```python
from build123d import *

# Parameters (mm, degrees)
F0_R     = 1.5875
F1_DEPTH = 1.6256


with BuildPart() as f1:
    # F0 (on Top) → F1 (new body)
    with BuildSketch(Plane.XY):
        with BuildLine():
            Line((-7.3025, -23.9776), (7.3025, -23.9776))
            ThreePointArc((7.3025, -23.9776), (8.425032, -23.512632), (8.89, -22.3901))
            Line((8.89, -22.3901), (8.89, 22.3901))
            ThreePointArc((8.89, 22.3901), (8.425032, 23.512632), (7.3025, 23.9776))
            Line((7.3025, 23.9776), (-7.3025, 23.9776))
            ThreePointArc((-7.3025, 23.9776), (-8.425032, 23.512632), (-8.89, 22.3901))
            Line((-8.89, 22.3901), (-8.89, -22.3901))
            ThreePointArc((-8.89, -22.3901), (-8.425032, -23.512632), (-7.3025, -23.9776))
        make_face()
        with Locations((0, -20.6756)):
            Circle(F0_R, mode=Mode.SUBTRACT)
        with Locations((0, 20.6756)):
            Circle(F0_R, mode=Mode.SUBTRACT)
    extrude(amount=-F1_DEPTH)


solid = f1.part
```
The listing builds one solid part. Answer for the finished solid, in the listing's coordinates (mm). Give positions to 0.01 mm unless a question says otherwise; leave off trailing zeros. Order: outer loops, then holes, each group sorted by start corner. A loop starts at its lowest first (then second) coordinate and runs counter-clockwise, first axis right, second up.
Item 1: For a pull along Y with two mould halves and no side action, classify faces 1 (the face through (-0.344, 19.126, -0.801)), 2 (the face through (0.853, -19.337, -0.801)), 3 (the face through (-8.89, 0, -1)), 4 (the face through (0, 23.978, -1)) as pulls with the +Y half, pulls with the -Y half, needs draft (parallel to the pull), parting line crosses it, or undercut.
From the geometry:
face 1: undercut
face 2: undercut
face 3: needs draft
face 4: pulls with the +Y half
Item 2: The part is cut by section A-A, the plane x = 0. Give the vertices of the cut face in (y, z).
From the geometry:
outline: (-23.98, -1.63) - (-22.26, -1.63) - (-22.26, 0) - (-23.98, 0) - close; (-19.09, -1.63) - (19.09, -1.63) - (19.09, 0) - (-19.09, 0) - close; (22.26, -1.63) - (23.98, -1.63) - (23.98, 0) - (22.26, 0) - close
Item 3: Given pin 1 Ø3 at (x, y) = (0, -20.68) entering from +Z, flat-ended and moving along its own axis, determine where the tip first touches the part or whether it passes through.
From the geometry:
pin 1: passes through
Item 4: The part is cut by section B-B, the plane z = -0.85. Give the vertices of the cut face in (x, y) (1 decimal), and give its area (3 significant figures).
From the geometry:
outline: (-8.9, -22.4) arc R1.6 ccw to (-7.3, -24) - (7.3, -24) arc R1.6 ccw to (8.9, -22.4) - (8.9, 22.4) arc R1.6 ccw to (7.3, 24) - (-7.3, 24) arc R1.6 ccw to (-8.9, 22.4) - close; hole circle Ø3.2 at (0, -20.7); hole circle Ø3.2 at (0, 20.7)
area: 835 mm2
Item 5: Find the intervals of material crossed by probe 1 along Y at (x, z) = (0, -0.6); probe 2 along X at (y, z) = (21.5, -0.25); probe 3 along X at (y, z) = (-21, -1.1), in increasing order.
From the geometry:
probe 1: y = -23.98 to -22.26, -19.09 to 19.09, 22.26 to 23.98
probe 2: x = -8.89 to -1.36, 1.36 to 8.89
probe 3: x = -8.89 to -1.55, 1.55 to 8.89
